Geometry: final body of the model. Coordinates: model frame, mm. A direction names the side the tool comes from. Coordinates: 2 decimals unless noted, no trailing zeros. Write each loop counter-clockwise with the first axis right and the second up, starting at its lowest first coordinate (ties: lowest second). Pieces come first, ordered by that corner, then holes. Notation, with made-up numbers: (-25, -24.75) -> (26, -24.75) arc R33 ccw to (26, 5.25) -> close; hole circle Ø5 at (-25.75, 83). An arc over 180 degrees is marked (long way). One line per item, written item: value.
```python
from build123d import *

# Parameters (mm, degrees)
SKETCH2_W                      = 38.1
SKETCH2_H                      = 38.1
BOSS_EXTRUDE1_DEPTH            = 2.54
F_5_16_0_3125_DIAMETER_HOLE1_D = 7.9375
BOSS_EXTRUDE2_DEPTH            = 2.54
F_10_0MM_DOWEL_HOLE1_D         = 10
MIRROR4_OUTLINE_R              = 5
MIRROR4_DEPTH                  = 2.54


# Read off the part's stored shape, not the designer's step: Mirror4
with BuildPart() as part:
    # Sketch2 → Boss-Extrude1 (new body)
    with BuildSketch(Plane.XY):
        with Locations((19.05, 19.05)):
            Rectangle(SKETCH2_W, SKETCH2_H)
    extrude(amount=BOSS_EXTRUDE1_DEPTH)

    # 5_16 _0.3125_ Diameter Hole1 (through all)
    with Locations(Plane(origin=(19.05, 19.05, 0), x_dir=(-1, 0, 0), z_dir=(0, 0, -1))):
        with Locations((0, 0)):
            Hole(F_5_16_0_3125_DIAMETER_HOLE1_D / 2)

    # Sketch4 → Boss-Extrude2 (add)
    with BuildSketch(Plane(origin=(0, 38.1, 0), x_dir=(1, 0, 0), z_dir=(0, 1, 0))):
        with BuildLine():
            Line((0, 0), (0, 16.51))
            ThreePointArc((0, 16.51), (5.207641431, 29.082358569), (17.78, 34.29))
            Line((17.78, 34.29), (20.32, 34.29))
            ThreePointArc((20.32, 34.29), (32.892358569, 29.082358569), (38.1, 16.51))
            Line((38.1, 16.51), (38.1, 0))
            Line((38.1, 0), (38.1, -2.54))
            Line((38.1, -2.54), (0, -2.54))
            Line((0, -2.54), (0, 0))
        make_face()
    extrude(amount=-BOSS_EXTRUDE2_DEPTH)

    # 10.0mm Dowel Hole1 (through all)
    with Locations(Plane(origin=(0, 38.1, 0), x_dir=(1, 0, 0), z_dir=(0, 1, 0))):
        with Locations((19.05, 21.59)):
            Hole(F_10_0MM_DOWEL_HOLE1_D / 2)

    # Mirror4 outline → Mirror4 (add)
    with BuildSketch(Plane(origin=(0, 0, 0), x_dir=(1, 0, 0), z_dir=(0, 1, 0))):
        with BuildLine():
            Line((0, 16.51), (0, 0))
            Line((0, 0), (38.1, 0))
            Line((38.1, 0), (38.1, 16.51))
            ThreePointArc((38.1, 16.51), (32.892358569, 29.082358569), (20.32, 34.29))
            Line((20.32, 34.29), (17.78, 34.29))
            ThreePointArc((17.78, 34.29), (5.207641431, 29.082358569), (0, 16.51))
        make_face()
        with Locations((19.05, 21.59)):
            Circle(MIRROR4_OUTLINE_R, mode=Mode.SUBTRACT)
    extrude(amount=MIRROR4_DEPTH)


solid = part.part
```
(1) Reachability of faces 1 (the flat face through (19, 2.54, -14)), 2 (the cylindrical face through (32.753, 36.848, -29.22)) from +Z, -Z, +X, -X, +Y, -Y: full face, straight path, thin tool, end or side. Return the list, or none.
Responses:
face 1: -Z, +X, -X
face 2: -Z, +X, +Y, -Y
(2) Pull-direction query (Y, two-part tool) for faces 3 (the cylindrical face through (14.055, 1.252, -21.81)), 4 (the flat face through (19, 35.56, -14)), 5 (the flat face through (19, 38.1, -16)), 6 (the flat face through (14.5, 19.3, 0)); classes: released by +Y, released by -Y, zero draft, split by the parting line, or undercut.
Responses:
face 3: zero draft
face 4: undercut
face 5: released by +Y
face 6: undercut
(3) Section B-B (z = -12.5). Return the cut outline in (x, y).
Responses:
outline: (0, 0) -> (38.1, 0) -> (38.1, 2.54) -> (0, 2.54) -> close; (0, 35.56) -> (38.1, 35.56) -> (38.1, 38.1) -> (0, 38.1) -> close
(4) Section A-A (y = 19.05). Return the cut outline in (x, z), then the cut area to 3 significant figures.
Responses:
outline: (0, 0) -> (15.08, 0) -> (15.08, 2.54) -> (0, 2.54) -> close; (23.02, 0) -> (38.1, 0) -> (38.1, 2.54) -> (23.02, 2.54) -> close
area: 76.6 mm2
(5) Section C-C (x = 19.05). Return the cut outline in (y, z), then the cut area to 3 significant figures.
Responses:
outline: (0, -34.29) -> (2.54, -34.29) -> (2.54, -26.59) -> (0, -26.59) -> close; (0, -16.59) -> (2.54, -16.59) -> (2.54, 0) -> (15.08, 0) -> (15.08, 2.54) -> (0, 2.54) -> close; (23.02, 0) -> (35.56, 0) -> (35.56, -16.59) -> (38.1, -16.59) -> (38.1, 2.54) -> (23.02, 2.54) -> close; (35.56, -34.29) -> (38.1, -34.29) -> (38.1, -26.59) -> (35.56, -26.59) -> close
area: 200 mm2
(6) Line query: line 1 (Y direction, x = 19, z = -27); line 2 (X direction, y = 19, z = 1); line 3 (Z direction, x = 19.05, y = 1). Output: solid intervals per line, ascending. Write a range as [from, to].
Responses:
line 1: y = [0, 2.54], [35.56, 38.1]
line 2: x = [0, 15.08], [23.02, 38.1]
line 3: z = [-34.29, -26.59], [-16.59, 2.54]
(7) Section D-D (z = -18.5). Return the cut outline in (x, y), then the cut area to 3 significant figures.
Responses:
outline: (0.11, 0) -> (15.12, 0) -> (15.12, 2.54) -> (0.11, 2.54) -> close; (0.11, 35.56) -> (15.12, 35.56) -> (15.12, 38.1) -> (0.11, 38.1) -> close; (22.98, 0) -> (37.99, 0) -> (37.99, 2.54) -> (22.98, 2.54) -> close; (22.98, 35.56) -> (37.99, 35.56) -> (37.99, 38.1) -> (22.98, 38.1) -> close
area: 152 mm2
(8) First-contact query: pin 1 (1 mm diameter, centred on x = 4, y = 28.5, fed in from -Z). Flat tip, straight axial feed; report the tip coordinate or a pass-through.
Responses:
pin 1: stops at z = 0
